```python
from build123d import *

# Parameters (mm, degrees)
SKETCH1_R           = 1
BOSS_EXTRUDE1_DEPTH = 1.7
SKETCH2_W           = 2
SKETCH2_H           = 2
BOSS_EXTRUDE2_DEPTH = 1
SKETCH3_W           = 7.9
SKETCH3_H           = 12
BOSS_EXTRUDE3_DEPTH = 5


with BuildPart() as part:
    # Sketch1 → Boss-Extrude1 (new body)
    with BuildSketch(Plane(origin=(0, 0, 0), x_dir=(1, 0, 0), z_dir=(0, 1, 0))):
        with BuildLine():
            Line((0, 0), (0, 8.2))
            ThreePointArc((0, 8.2), (-1.8, 10), (0, 11.8))
            Line((0, 11.8), (0, 20))
            Line((0, 20), (5.5, 20))
            ThreePointArc((5.5, 20), (8, 17.5), (10.5, 20))
            Line((10.5, 20), (28.2, 20))
            ThreePointArc((28.2, 20), (30, 21.8), (31.8, 20))
            Line((31.8, 20), (40, 20))
            Line((40, 20), (40, 16))
            Line((40, 16), (38, 16))
            Line((38, 16), (38, 4))
            Line((38, 4), (40, 4))
            Line((40, 4), (40, 0))
            Line((40, 0), (31.8, 0))
            ThreePointArc((31.8, 0), (30, -1.8), (28.2, 0))
            Line((28.2, 0), (10.5, 0))
            ThreePointArc((10.5, 0), (8, 2.5), (5.5, 0))
            Line((5.5, 0), (0, 0))
        make_face()
        with Locations((0, 10)):
            Circle(SKETCH1_R, mode=Mode.SUBTRACT)
        with Locations((30, 0)):
            Circle(SKETCH1_R, mode=Mode.SUBTRACT)
        with Locations((30, 20)):
            Circle(SKETCH1_R, mode=Mode.SUBTRACT)
        Polygon((4.3, 14.5), (11.3, 14.5), (11.3, 13.5), (5.3, 13.5), (5.3, 6.5), (11.3, 6.5), (11.3, 5.5), (4.3, 5.5), align=None, mode=Mode.SUBTRACT)
    extrude(amount=BOSS_EXTRUDE1_DEPTH)

    # Sketch2 → Boss-Extrude2 (add)
    with BuildSketch(Plane(origin=(0, 1.7, 0), x_dir=(1, 0, 0), z_dir=(0, 1, 0))):
        with Locations((7.3, 10)):
            Rectangle(SKETCH2_W, SKETCH2_H)
    extrude(amount=BOSS_EXTRUDE2_DEPTH)

    # Sketch3 → Boss-Extrude3 (add)
    with BuildSketch(Plane(origin=(0, 1.7, 0), x_dir=(1, 0, 0), z_dir=(0, 1, 0))):
        with Locations((34.05, 10)):
            Rectangle(SKETCH3_W, SKETCH3_H)
    extrude(amount=BOSS_EXTRUDE3_DEPTH)


solid = part.part
```
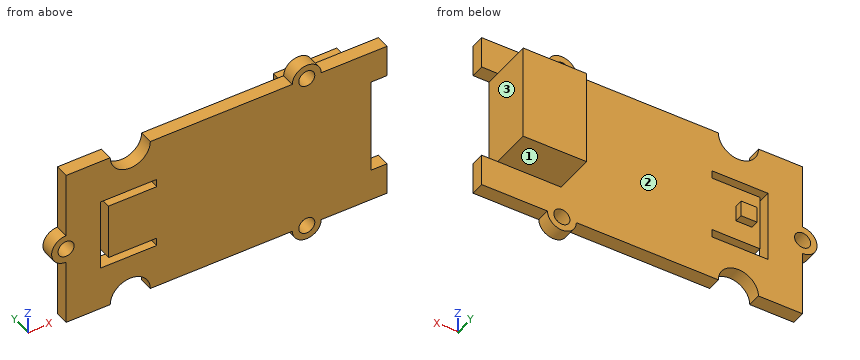
Source: CAD feature listing. Evaluate the final solid. Frame: model axes, mm. Face numbers are marked on the shaded views. Round coordinates to 2 decimals unless told otherwise and drop trailing zeros. Loops run counter-clockwise (first coordinate to the right, second up) from the corner with the lowest first, then second, coordinate; pieces in that order, holes last.
(1) Pull-direction query (Z, two-part tool) for the marked faces 1, 2 and 3; classes: +Z half, -Z half, draft (parallel to the pull), parting line (faces both ways), or undercut.
From the geometry:
face 1: -Z half
face 2: draft
face 3: undercut
(2) Section query A-A (z = -10). Output: boundary loops of the cut face in (x, y).
From the geometry:
outline: (-1.8, 0) - (-1, 0) - (-1, 1.7) - (-1.8, 1.7) - close; (1, 0) - (4.3, 0) - (4.3, 1.7) - (1, 1.7) - close; (5.3, 0) - (38, 0) - (38, 6.7) - (30.1, 6.7) - (30.1, 1.7) - (8.3, 1.7) - (8.3, 2.7) - (6.3, 2.7) - (6.3, 1.7) - (5.3, 1.7) - close
(3) Material intervals for probe 1 along Z at (x, y) = (30, 1); probe 2 along Y at (x, z) = (36.5, -17.75); probe 3 along X at (y, z) = (2.25, -14), sorted ascending.
From the geometry:
probe 1: z = -21.8 to -21, -19 to -1, 1 to 1.8
probe 2: y = 0 to 1.7
probe 3: x = 30.1 to 38
(4) Section query B-B (y = 3.25). Output: boundary loops of the cut face in (x, z), and give its area (3 significant figures).
From the geometry:
outline: (30.1, -16) - (38, -16) - (38, -4) - (30.1, -4) - close
area: 94.8 mm2
(5) Section query C-C (z = -5). Output: boundary loops of the cut face in (x, y), and give its area (3 significant figures).
From the geometry:
outline: (0, 0) - (38, 0) - (38, 6.7) - (30.1, 6.7) - (30.1, 1.7) - (0, 1.7) - close
area: 104 mm2
(6) Contact query for flat-ended pins moving along their axis: pin 1 Ø1.4 at (x, y) = (8.5, 1) entering from +Z; pin 2 Ø3 at (x, y) = (11, 4.5) entering from -Z; pin 3 Ø1.1 at (y, z) = (2, -9.5) entering from +X; pin 4 Ø0.5 at (x, y) = (17, 1) entering from +Z. Output: stop coordinate, or through.
From the geometry:
pin 1: stops at z = -2.19
pin 2: passes through
pin 3: stops at x = 38
pin 4: stops at z = 0
